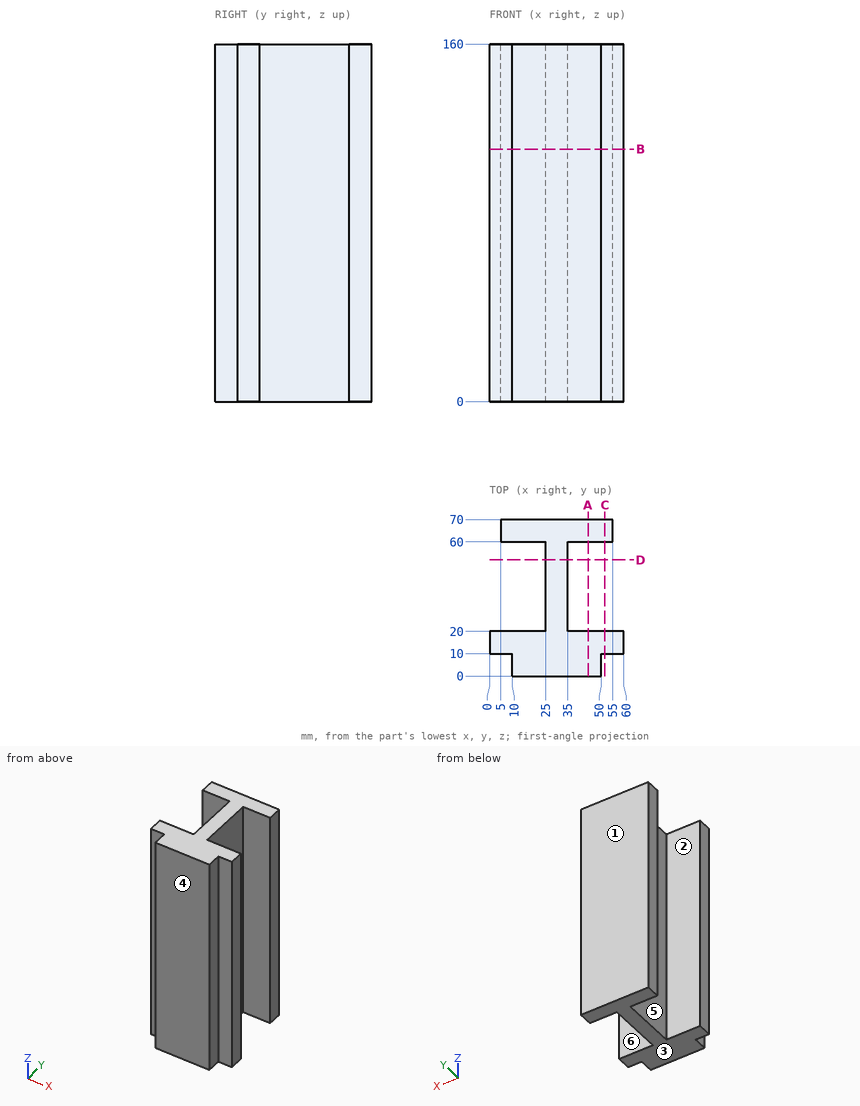
Job drawing, mm, ordinate dimensions from the low corner. One solid piece. A direction names the side the tool comes from. Coordinates: 2 decimals unless noted, no trailing zeros. Write each loop counter-clockwise with the first axis right and the second up, starting at its lowest first coordinate (ties: lowest second). Pieces come first, ordered by that corner, then holes. Notation, with made-up numbers: (86.5, 74) - (138.5, 74) arc R24 cw to (138.5, 88) - close; hole circle Ø11 at (27, -10.5). An arc over 180 degrees is marked (long way). Use a Markdown table: item, result. Add a question column.
Item 1: Drill centre lines: L1, parallel to Y at x = 13.5, z = 101; L2, parallel to Y at x = 53, z = 144; L3, parallel to X at y = 54, z = 97. Where is each one in solid material? Low to high. Write a range as from..to.
Item 2: Flat gauge pins, fed straight in: pin 1 (3 mm diameter, centred on y = 67, z = 65, fed in from +X); pin 2 (3 mm diameter, centred on x = 56.5, z = 57.5, fed in from -Y); pin 3 (11 mm diameter, centred on y = 2.5, z = 53, fed in from -X). Where does each tip first touch, or does it go through?
Item 3: 3-axis set-ups, long thin cutter, end or side, ignore diameter. For the marked faces 4, 5 and 6: which of +Z, -Z, +X, -X, +Y, -Y reach the whole face in a straight line?
Item 4: Band-saw the part on D-D, the plane y = 52. Give the cut face in (x, z).
Item 5: Band-saw the part on B-B, the plane z = 113. Give the cut face in (x, y), and give its area (3 significant figures).
Item 6: Mould opens along Y. For the marked faces 1, 2 and 3 say: pulls with the +Y half, pulls with the -Y half, needs draft (parallel to the pull), parting line crosses it, or undercut.
Item 7: Band-saw the part on A-A, the plane x = 44. Give the cut face in (y, z), and give its area (3 significant figures).
Item 8: Band-saw the part on C-C, the plane x = 51.5. Give the cut face in (y, z), and give its area (3 significant figures).
Numbers:
| question | item | result |
|---|---|---|
| 1 | L1 | 0..20, 60..70 |
| 1 | L2 | 10..20, 60..70 |
| 1 | L3 | 25..35 |
| 2 | pin 1 | x = 55 |
| 2 | pin 2 | y = 10 |
| 2 | pin 3 | x = 10 |
| 3 | face 4 | +Z, -Z, +X, -X, -Y |
| 3 | face 5 | +Z, -Z, -X |
| 3 | face 6 | +Z, -Z, +X |
| 4 | outline | (25, 0) - (35, 0) - (35, 160) - (25, 160) - close |
| 5 | outline | (0, 10) - (10, 10) - (10, 0) - (50, 0) - (50, 10) - (60, 10) - (60, 20) - (35, 20) - (35, 60) - (55, 60) - (55, 70) - (5, 70) - (5, 60) - (25, 60) - (25, 20) - (0, 20) - close |
| 5 | area | 1,900 mm2 |
| 6 | face 1 | pulls with the +Y half |
| 6 | face 2 | undercut |
| 6 | face 3 | needs draft |
| 7 | outline | (0, 0) - (20, 0) - (20, 160) - (0, 160) - close; (60, 0) - (70, 0) - (70, 160) - (60, 160) - close |
| 7 | area | 4,800 mm2 |
| 8 | outline | (10, 0) - (20, 0) - (20, 160) - (10, 160) - close; (60, 0) - (70, 0) - (70, 160) - (60, 160) - close |
| 8 | area | 3,200 mm2 |
